Build history of the part. All positions in model axes, mm. Face numbers are marked on the shaded views. A direction names the side the tool comes from. Give positions to 0.01 mm unless a question says otherwise; leave off trailing zeros. Write each loop counter-clockwise with the first axis right and the second up, starting at its lowest first coordinate (ties: lowest second). Pieces come first, ordered by that corner, then holes.
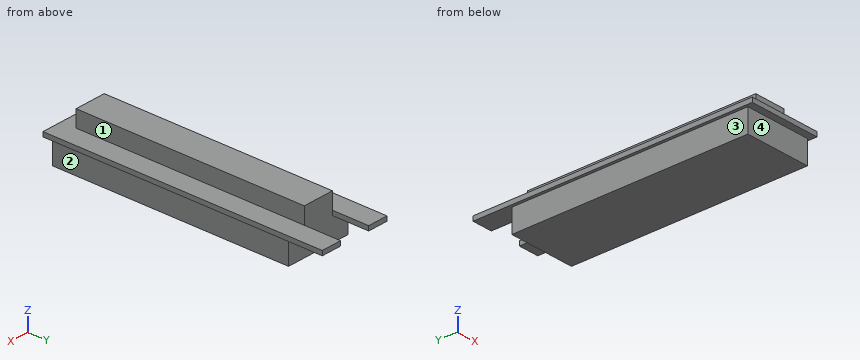
from build123d import *

# Parameters (mm, degrees)
F1_DEPTH = 1.25
F2_W     = 8.7
F2_H     = 62.917138
F3_DEPTH = 5.8
F5_DEPTH = 6.4


with BuildPart() as f1:
    # F0 (on Top) → F1 (new body)
    with BuildSketch(Plane.XY):
        Polygon((-10, -38.5), (10, -38.5), (10, 38.5), (4.35, 38.5), (4.35, 28.5), (-4.35, 28.5), (-4.35, 38.5), (-10, 38.5), align=None)
    extrude(amount=F1_DEPTH)

    # F2 (on face) → F3 (join)
    with BuildSketch(Plane(origin=(0, 0, 0), x_dir=(1, 0, 0), z_dir=(0, 0, -1))):
        with Locations((0, 2.958569)):
            Rectangle(F2_W, F2_H)
    extrude(amount=-F3_DEPTH)

    # F4 (on face) → F5 (join)
    with BuildSketch(Plane(origin=(0, 0, 0), x_dir=(1, 0, 0), z_dir=(0, 0, -1))):
        Polygon((-9.20814, 36.568932), (-9.20814, -28.5), (-4.35, -28.5), (4.35, -28.5), (9.20814, -28.5), (9.20814, 36.568932), align=None)
    extrude(amount=F5_DEPTH)


solid = f1.part
1. Saw through at B-B on y = -9. Give the cut face in (x, z), plus the area to 3 significant figures.
2. Saw through at C-C on z = 4.5. Give the cut face in (x, y), plus the area to 3 significant figures.
3. Saw through at A-A on x = -6.25. Give the cut face in (y, z), plus the area to 3 significant figures.
4. Saw through at D-D on x = 2.75. Give the cut face in (y, z), plus the area to 3 significant figures.
5. 3-axis set-ups, long thin cutter, end or side, ignore diameter. For the marked faces 1, 2, 3 and 4: which of +Z, -Z, +X, -X, +Y, -Y reach the whole face in a straight line?
6. Drill centre lines: line 1 along Z through (x, y) = (9, -9.5); line 2 along Y through (x, z) = (4.5, -5); line 3 along X through (y, z) = (26.5, 3.25). Where is each one in solid material? Low to high.
7. Drop flat-ended pins along their axis: pin 1 (3.5 mm diameter, centred on y = -2, z = 3.5, fed in from +X); pin 2 (6 mm diameter, centred on y = -3.5, z = -4, fed in from -X); pin 3 (1 mm diameter, centred on y = -8, z = -5, fed in from +X). Give the stop position or say it passes through.
Outcome:
1. outline: (-10, 0) - (-9.21, 0) - (-9.21, -6.4) - (9.21, -6.4) - (9.21, 0) - (10, 0) - (10, 1.25) - (4.35, 1.25) - (4.35, 5.8) - (-4.35, 5.8) - (-4.35, 1.25) - (-10, 1.25) - close
1. area: 182 mm2
2. outline: (-4.35, -34.42) - (4.35, -34.42) - (4.35, 28.5) - (-4.35, 28.5) - close
2. area: 547 mm2
3. outline: (-38.5, 0) - (-36.57, 0) - (-36.57, -6.4) - (28.5, -6.4) - (28.5, 0) - (38.5, 0) - (38.5, 1.25) - (-38.5, 1.25) - close
3. area: 513 mm2
4. outline: (-38.5, 0) - (-36.57, 0) - (-36.57, -6.4) - (28.5, -6.4) - (28.5, 5.8) - (-34.42, 5.8) - (-34.42, 1.25) - (-38.5, 1.25) - close
4. area: 786 mm2
5. face 1: +Z, +X, +Y, -Y
5. face 2: -Z, +X, +Y, -Y
5. face 3: -Z, -X, +Y, -Y
5. face 4: -Z, +X, -X, -Y
6. line 1: z = -6.4 to 1.25
6. line 2: y = -36.57 to 28.5
6. line 3: x = -4.35 to 4.35
7. pin 1: stops at x = 4.35
7. pin 2: stops at x = -9.21
7. pin 3: stops at x = 9.21
